Drawing for the job (mm, zero at the part's lowest x, y, z). A direction names the side the tool comes from. Coordinates: 2 decimals unless noted, no trailing zeros. Loops run counter-clockwise (first coordinate to the right, second up) from the corner with the lowest first, then second, coordinate; pieces in that order, holes last. Notation, with made-up numbers: (-15.75, 4.25) - (15.25, 4.25) arc R35 cw to (15.25, 36.25) - close; hole circle Ø6 at (38.25, 32.5). An arc over 180 degrees is marked (long way). One line per item, written item: value.
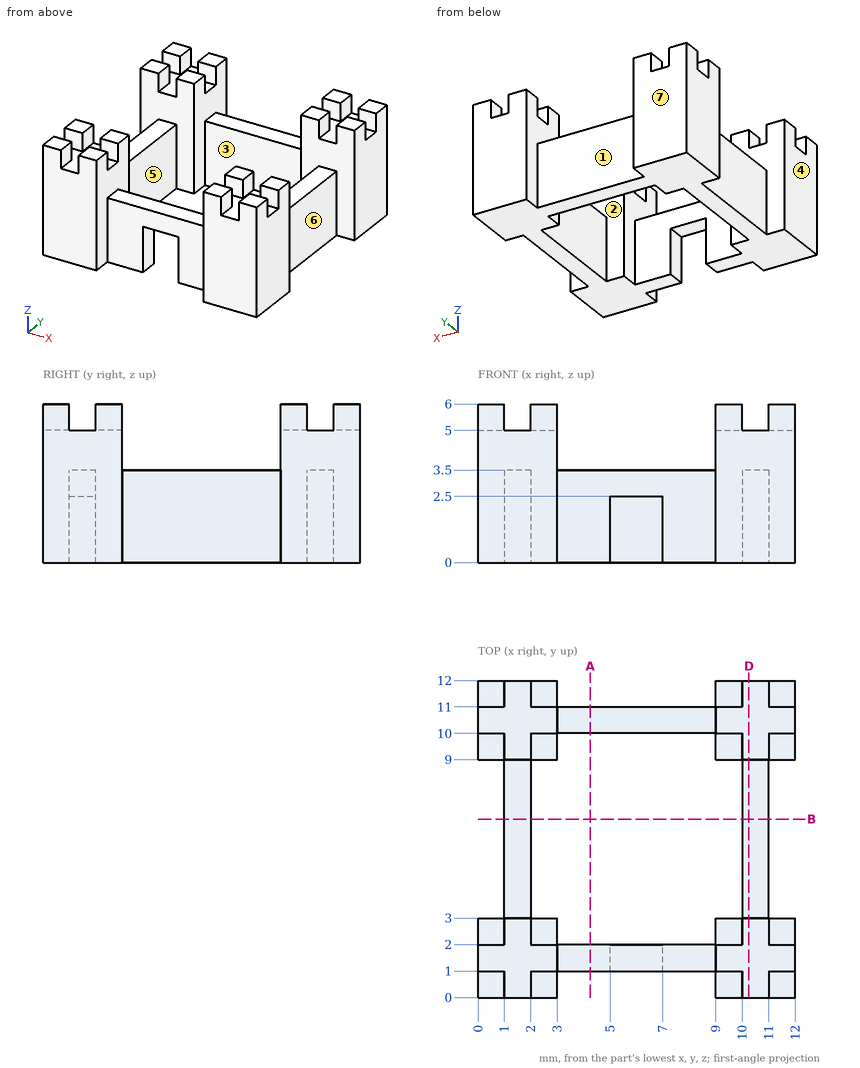
Item 1: Drop flat-ended pins along their axis: P1, Ø3, axis at x = 9.5, z = 5.5, coming from the -Y side; P2, Ø1.8, axis at y = 6, z = 1, coming from the -X side; P3, Ø1.1, axis at x = 1.5, y = 7.5, coming from the +Z side; P4, Ø1.8, axis at y = 6, z = 2, coming from the +X side. Give the stop position or say it passes through.
Check result:
P1: stops at y = 0
P2: stops at x = 1
P3: stops at z = 3.5
P4: stops at x = 11
Item 2: Cut at A-A, the plane x = 4.25. Write the cut outline in (y, z).
Check result:
outline: (1, 0) - (2, 0) - (2, 3.5) - (1, 3.5) - close; (10, 0) - (11, 0) - (11, 3.5) - (10, 3.5) - close
Item 3: Probe probe 1 along Y at (x, z) = (2.25, 5.6); probe 2 along Y at (x, z) = (9.75, 2.9); probe 3 along Y at (x, z) = (4, 1.35). List the from-to ranges inside material, lowest first. Write a range as from..to.
Check result:
probe 1: y = 0..1, 2..3, 9..10, 11..12
probe 2: y = 0..3, 9..12
probe 3: y = 1..2, 10..11
Item 4: Tool access for the marked faces 1, 2 and 3: list every direction of +Z, -Z, +X, -X, +Y, -Y with a clear straight run to the whole face (end or side of a thin tool).
Check result:
face 1: +Z, -Z, +Y
face 2: +Z
face 3: +Z, -Z
Item 5: Cut at D-D, the plane x = 10.25. Write the cut outline in (y, z), then the cut area to 3 significant figures.
Check result:
outline: (0, 0) - (12, 0) - (12, 5) - (9, 5) - (9, 3.5) - (3, 3.5) - (3, 5) - (0, 5) - close
area: 51.0 mm^2
Item 6: Pull direction X, two halves, no side cores. Call the marked faces 4, 5, 6 and 7: released by +X, released by -X, zero draft, split by the parting line, or undercut.
Check result:
face 4: released by -X
face 5: undercut
face 6: released by +X
face 7: zero draft
